Here's the drawing with two shaded views (mm, measured from the low corner). I have some questions. A direction names the side the tool comes from. Give positions to 0.01 mm unless a question says otherwise; leave off trailing zeros. Write each loop counter-clockwise with the first axis right and the second up, starting at its lowest first coordinate (ties: lowest second). Pieces come first, ordered by that corner, then holes. Notation, with made-up numbers: (34.5, -5) -> (62.5, -5) arc R25 ccw to (62.5, 33) -> close; hole circle Ø8 at (63.5, 55). An arc over 180 degrees is marked (long way). One line per item, written item: value.
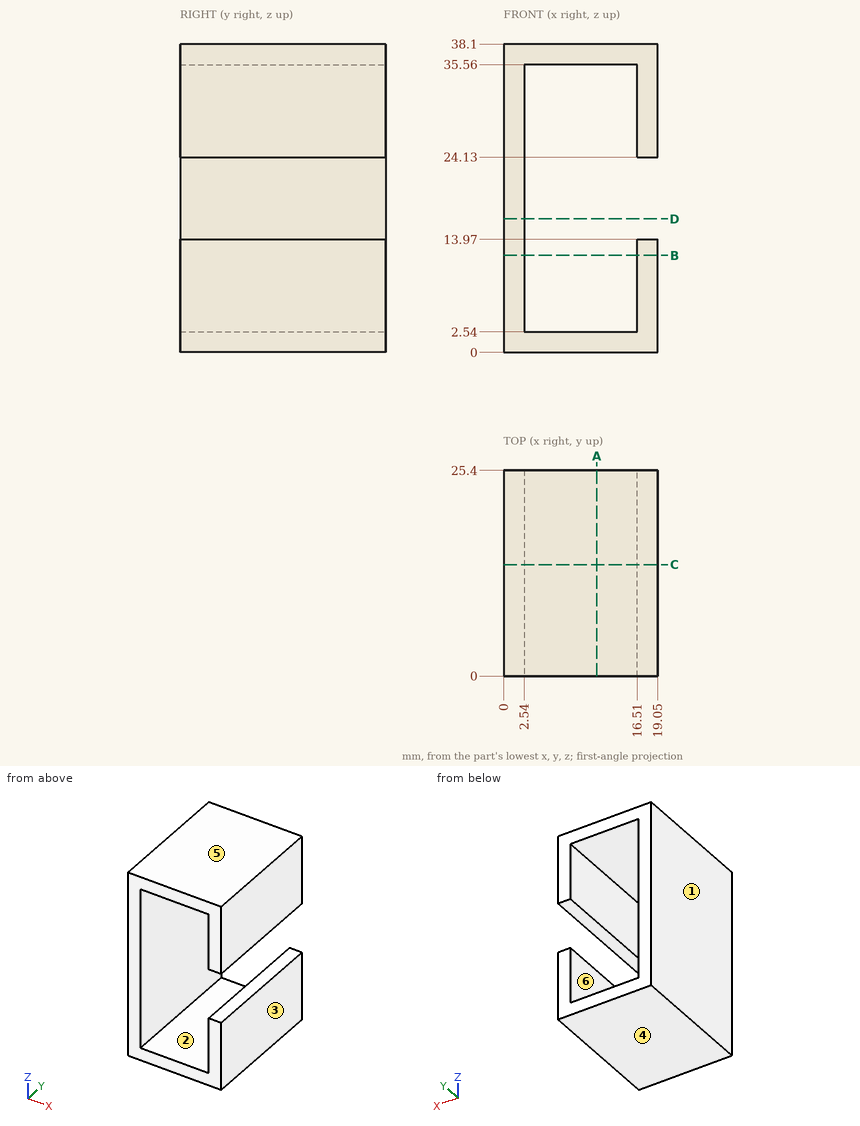
1) If we section it at B-B (z = 12): Write out the boundary of the cut face in (x, y).
Answer list:
outline: (0, 0) -> (2.54, 0) -> (2.54, 25.4) -> (0, 25.4) -> close; (16.51, 0) -> (19.05, 0) -> (19.05, 25.4) -> (16.51, 25.4) -> close
2) For the marked faces 1 and 2, which set-ups out of +Z, -Z, +X, -X, +Y, -Y let a thin tool reach every point of the face, with its end or its side?
Answer list:
face 1: +Z, -Z, -X, +Y, -Y
face 2: +Y, -Y
3) If we section it at A-A (x = 11.5): Write out the boundary of the cut face in (y, z), and give its area (3 significant figures).
Answer list:
outline: (0, 0) -> (25.4, 0) -> (25.4, 2.54) -> (0, 2.54) -> close; (0, 35.56) -> (25.4, 35.56) -> (25.4, 38.1) -> (0, 38.1) -> close
area: 129 mm^2
4) I need wall thicknesses on L1, parallel to Z at x = 4, y = 8.25; L2, parallel to X at y = 11, z = 12; L3, parallel to X at y = 8, z = 15.5. Which ranges of each line are inside material? Lowest first, please.
Answer list:
L1: z = 0 to 2.54, 35.56 to 38.1
L2: x = 0 to 2.54, 16.51 to 19.05
L3: x = 0 to 2.54
5) We'd pull the mould along Z, two halves only. Please class the marked faces 3, 4, 5 and 6: released by +Z, released by -Z, zero draft, split by the parting line, or undercut.
Answer list:
face 3: zero draft
face 4: released by -Z
face 5: released by +Z
face 6: undercut
6) Will this pin go through, and if not, where does the flat tip stop? pin 1 (1 mm diameter, centred on y = 13, z = 20, fed in from +X).
Answer list:
pin 1: stops at x = 2.54
7) If we section it at D-D (z = 16.5): Write out the boundary of the cut face in (x, y).
Answer list:
outline: (0, 0) -> (2.54, 0) -> (2.54, 25.4) -> (0, 25.4) -> close
8) If we section it at C-C (y = 13.75): Write out the boundary of the cut face in (x, z).
Answer list:
outline: (0, 0) -> (19.05, 0) -> (19.05, 13.97) -> (16.51, 13.97) -> (16.51, 2.54) -> (2.54, 2.54) -> (2.54, 35.56) -> (16.51, 35.56) -> (16.51, 24.13) -> (19.05, 24.13) -> (19.05, 38.1) -> (0, 38.1) -> close
